```python
from build123d import *

# Parameters (mm, degrees)
BOSS_EXTRUDE1_DEPTH = 3
SKETCH1_3_R         = 8
BOSS_EXTRUDE2_DEPTH = 6
SKETCH1_5_R         = 8
SKETCH1_5_R_2       = 3.3
BOSS_EXTRUDE4_DEPTH = 18


with BuildPart() as part:
    # Sketch1 → Boss-Extrude1 (new body)
    with BuildSketch(Plane.XY):
        with BuildLine():
            ThreePointArc((42.894958583, -3.003752345), (43.557934635, -6.502479184), (45.856433127, -9.222319513))
            ThreePointArc((45.856433127, -9.222319513), (50.229473419, -29), (30.914979544, -35.101676259))
            ThreePointArc((30.914979544, -35.101676259), (27.410279478, -34.471038339), (24.048805129, -35.646247655))
            ThreePointArc((24.048805129, -35.646247655), (0, -43), (-24.048805129, -35.646247655))
            ThreePointArc((-24.048805129, -35.646247655), (-27.410279478, -34.471038339), (-30.914979544, -35.101676259))
            ThreePointArc((-30.914979544, -35.101676259), (-50.229473419, -29), (-45.856433127, -9.222319513))
            ThreePointArc((-45.856433127, -9.222319513), (-43.557934635, -6.502479184), (-42.894958583, -3.003752345))
            ThreePointArc((-42.894958583, -3.003752345), (-37.239092363, 21.5), (-18.846153454, 38.65))
            ThreePointArc((-18.846153454, 38.65), (-16.147655157, 40.973517522), (-14.941453584, 44.323995772))
            ThreePointArc((-14.941453584, 44.323995772), (0, 58), (14.941453584, 44.323995772))
            ThreePointArc((14.941453584, 44.323995772), (16.147655157, 40.973517523), (18.846153454, 38.65))
            ThreePointArc((18.846153454, 38.65), (37.239092363, 21.5), (42.894958583, -3.003752345))
        make_face()
        with BuildLine():
            ThreePointArc((39.902287054, -2.794188228), (34.641016151, 20), (17.531305538, 35.953488372))
            ThreePointArc((17.531305538, 35.953488372), (13.676307972, 39.272799119), (11.953162867, 44.059196617))
            ThreePointArc((11.953162867, 44.059196617), (0, 55), (-11.953162867, 44.059196617))
            ThreePointArc((-11.953162867, 44.059196617), (-13.676307972, 39.272799119), (-17.531305538, 35.953488372))
            ThreePointArc((-17.531305538, 35.953488372), (-34.641016151, 20), (-39.902287054, -2.794188228))
            ThreePointArc((-39.902287054, -2.794188228), (-40.8493957, -7.792369426), (-44.132964974, -11.67785561))
            ThreePointArc((-44.132964974, -11.67785561), (-47.631397208, -27.5), (-32.179802107, -32.381341007))
            ThreePointArc((-32.179802107, -32.381341007), (-27.173087728, -31.480429693), (-22.370981516, -33.159300144))
            ThreePointArc((-22.370981516, -33.159300144), (0, -40), (22.370981516, -33.159300144))
            ThreePointArc((22.370981516, -33.159300144), (27.173087728, -31.480429693), (32.179802107, -32.381341007))
            ThreePointArc((32.179802107, -32.381341007), (47.631397208, -27.5), (44.132964974, -11.67785561))
            ThreePointArc((44.132964974, -11.67785561), (40.8493957, -7.792369426), (39.902287054, -2.794188228))
        make_face(mode=Mode.SUBTRACT)
    extrude(amount=BOSS_EXTRUDE1_DEPTH)

    # Sketch1_3 → Boss-Extrude2 (add)
    with BuildSketch(Plane.XY):
        with BuildLine():
            ThreePointArc((39.902287054, -2.794188228), (40.8493957, -7.792369426), (44.132964974, -11.67785561))
            ThreePointArc((44.132964974, -11.67785561), (47.631397208, -27.5), (32.179802107, -32.381341007))
            ThreePointArc((32.179802107, -32.381341007), (27.173087728, -31.480429693), (22.370981516, -33.159300144))
            ThreePointArc((22.370981516, -33.159300144), (0, -40), (-22.370981516, -33.159300144))
            ThreePointArc((-22.370981516, -33.159300144), (-27.173087728, -31.480429693), (-32.179802107, -32.381341007))
            ThreePointArc((-32.179802107, -32.381341007), (-47.631397208, -27.5), (-44.132964974, -11.67785561))
            ThreePointArc((-44.132964974, -11.67785561), (-40.8493957, -7.792369426), (-39.902287054, -2.794188228))
            ThreePointArc((-39.902287054, -2.794188228), (-34.641016151, 20), (-17.531305538, 35.953488372))
            ThreePointArc((-17.531305538, 35.953488372), (-13.676307972, 39.272799119), (-11.953162867, 44.059196617))
            ThreePointArc((-11.953162867, 44.059196617), (0, 55), (11.953162867, 44.059196617))
            ThreePointArc((11.953162867, 44.059196617), (13.676307972, 39.272799119), (17.531305538, 35.953488372))
            ThreePointArc((17.531305538, 35.953488372), (34.641016151, 20), (39.902287054, -2.794188228))
        make_face()
        with Locations((-37.239092363, -21.5)):
            Circle(SKETCH1_3_R, mode=Mode.SUBTRACT)
        with Locations((37.239092363, -21.5)):
            Circle(SKETCH1_3_R, mode=Mode.SUBTRACT)
        with Locations((0, 43)):
            Circle(SKETCH1_3_R, mode=Mode.SUBTRACT)
    extrude(amount=BOSS_EXTRUDE2_DEPTH)

    # Sketch1_5 → Boss-Extrude4 (add)
    # profile 1 of 3: a face of its own
    with BuildSketch(Plane.XY):
        with Locations((37.239092363, -21.5)):
            Circle(SKETCH1_5_R)
        with Locations((37.239092363, -21.5)):
            Circle(SKETCH1_5_R_2, mode=Mode.SUBTRACT)
    # profile 2 of 3: a face of its own
    with BuildSketch(Plane.XY):
        with Locations((-37.239092363, -21.5)):
            Circle(SKETCH1_5_R)
        with Locations((-37.239092363, -21.5)):
            Circle(SKETCH1_5_R_2, mode=Mode.SUBTRACT)
    # profile 3 of 3: a face of its own
    with BuildSketch(Plane.XY):
        with Locations((0, 43)):
            Circle(SKETCH1_5_R)
        with Locations((0, 43)):
            Circle(SKETCH1_5_R_2, mode=Mode.SUBTRACT)
    extrude(amount=BOSS_EXTRUDE4_DEPTH)


solid = part.part
```
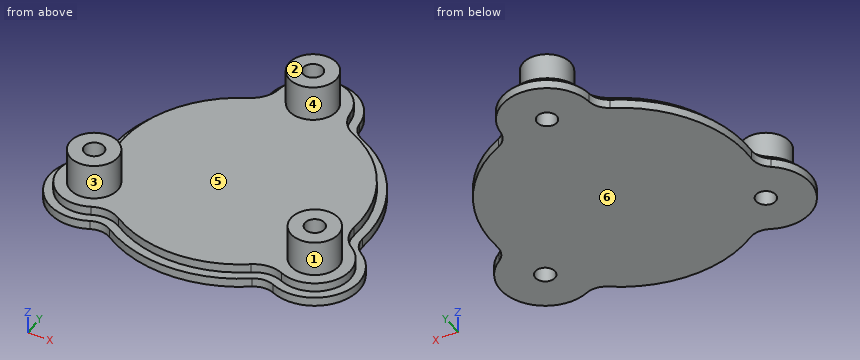
Source: CAD feature listing. Evaluate the final solid. Frame: model axes, mm. Face numbers are marked on the shaded views. A direction names the side the tool comes from. Round coordinates to 2 decimals unless told otherwise and drop trailing zeros. Loops run counter-clockwise (first coordinate to the right, second up) from the corner with the lowest first, then second, coordinate; pieces in that order, holes last.
(1) Access query for the marked faces 5 and 6. Directions: +Z, -Z, +X, -X, +Y, -Y. A direction counts if a zero-diameter tool reaches every point of the face in a straight line with its end or side. Return the directions, or none.
From the geometry:
face 5: +Z
face 6: -Z, +X, -X, +Y, -Y
(2) Section query B-B (x = 0). Output: boundary loops of the cut face in (y, z), and give its area (3 significant figures).
From the geometry:
outline: (-43, 0) - (39.7, 0) - (39.7, 18) - (35, 18) - (35, 6) - (-40, 6) - (-40, 3) - (-43, 3) - close; (46.3, 0) - (58, 0) - (58, 3) - (55, 3) - (55, 6) - (51, 6) - (51, 18) - (46.3, 18) - close
area: 661 mm2
(3) Contact query for flat-ended pins moving along their axis: pin 1 Ø6 at (y, z) = (44.5, 2.5) entering from -X; pin 2 Ø3 at (y, z) = (20, 5) entering from +X; pin 3 Ø4 at (x, y) = (20.5, 13.5) entering from +Z. Output: stop coordinate, or through.
From the geometry:
pin 1: stops at x = -15.82
pin 2: stops at x = 35.46
pin 3: stops at z = 6
(4) Section query D-D (z = 1.75). Output: boundary loops of the cut face in (x, y).
From the geometry:
outline: (-45.86, -9.22) arc R15 ccw to (-30.91, -35.1) arc R7 cw to (-24.05, -35.65) arc R43 ccw to (24.05, -35.65) arc R7 cw to (30.91, -35.1) arc R15 ccw to (45.86, -9.22) arc R7 cw to (42.89, -3) arc R43 ccw to (18.85, 38.65) arc R7 cw to (14.94, 44.32) arc R15 ccw to (-14.94, 44.32) arc R7 cw to (-18.85, 38.65) arc R43 ccw to (-42.89, -3) arc R7 cw to start; hole circle Ø6.6 at (-37.24, -21.5); hole circle Ø6.6 at (0, 43); hole circle Ø6.6 at (37.24, -21.5)
(5) Material intervals for probe 1 along Y at (x, z) = (0, 9.5); probe 2 along Z at (x, y) = (21, -15.5); probe 3 along Y at (x, z) = (-38.5, 1.5), sorted ascending.
From the geometry:
probe 1: y = 35 to 39.7, 46.3 to 51
probe 2: z = 0 to 6
probe 3: y = -36.45 to -24.55, -18.45 to 19.15
(6) Section query C-C (y = -21.5). Output: boundary loops of the cut face in (x, z), and give its area (3 significant figures).
From the geometry:
outline: (-52.24, 0) - (-40.54, 0) - (-40.54, 18) - (-45.24, 18) - (-45.24, 6) - (-49.24, 6) - (-49.24, 3) - (-52.24, 3) - close; (-33.94, 0) - (33.94, 0) - (33.94, 18) - (29.24, 18) - (29.24, 6) - (-29.24, 6) - (-29.24, 18) - (-33.94, 18) - close; (40.54, 0) - (52.24, 0) - (52.24, 3) - (49.24, 3) - (49.24, 6) - (45.24, 6) - (45.24, 18) - (40.54, 18) - close
area: 755 mm2
(7) Pull-direction query (X, two-part tool) for the marked faces 1, 2, 3 and 4; classes: +X half, -X half, draft (parallel to the pull), parting line (faces both ways), or undercut.
From the geometry:
face 1: undercut
face 2: draft
face 3: undercut
face 4: parting line
(8) Section query A-A (z = 7.5). Output: boundary loops of the cut face in (x, y), and give its area (3 significant figures).
From the geometry:
outline: circle Ø16 at (-37.24, -21.5); circle Ø16 at (0, 43); circle Ø16 at (37.24, -21.5); hole circle Ø6.6 at (-37.24, -21.5); hole circle Ø6.6 at (0, 43); hole circle Ø6.6 at (37.24, -21.5)
area: 501 mm2
